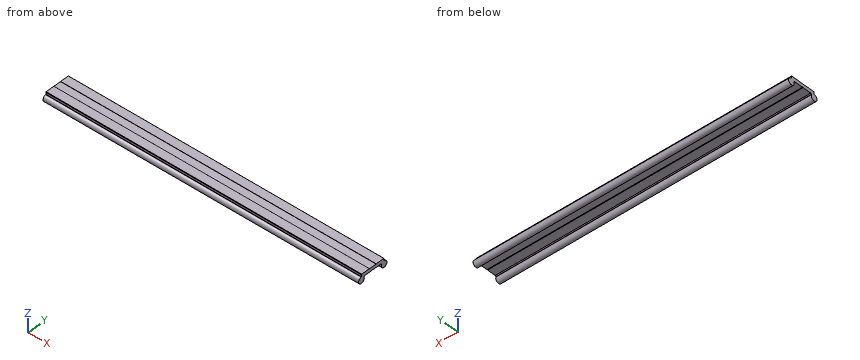
Autodesk Inventor part; units mm, degrees
ref_plane "YZ Plane" through (0, 0, 0) normal (1, 0, 0) x (0, 1, 0)
ref_plane "XZ Plane" through (0, 0, 0) normal (0, 1, 0) x (-1, 0, 0)
ref_plane "XY Plane" through (0, 0, 0) normal (0, 0, 1) x (1, 0, 0)
sketch "Szkic1" plane through (0, 0, 0) normal (1, 0, 0) x (0, 1, 0)
  line L0 (13.7, -0.2) -> (25.3, -0.2)
  line L1 (13.5, 0) -> (13.7, -0.2)
  line L2 (0, 0) -> (13.5, 0)
  line L3 (-0.5, -0.5) -> (0, 0)
  line L4 (-0.5, -3.7085) -> (-0.5, -0.5)
  arc A0 (-0.783, -4.008) -> (-0.5, -3.7085) centre (-0.8, -3.7085) ccw
  arc A1 (-0.783, -4.008) -> (3.9514, -6.7229) centre (-0.5, -9) ccw
  arc A2 (4.0685, -6.3265) -> (3.9514, -6.7229) centre (4.2185, -6.5863) ccw
  line L5 (5.5, -5.5) -> (4.0685, -6.3265)
  line L6 (19, -5.5) -> (5.5, -5.5)
  line L7 (19.5, -5.2113) -> (19, -5.5)
  line L8 (20, -5.5) -> (19.5, -5.2113)
  line L9 (33.5, -5.5) -> (20, -5.5)
  line L10 (34.9315, -6.3265) -> (33.5, -5.5)
  arc A3 (35.0486, -6.7229) -> (34.9315, -6.3265) centre (34.7815, -6.5863) ccw
  arc A4 (35.0486, -6.7229) -> (39.783, -4.008) centre (39.5, -9) ccw
  arc A5 (39.5, -3.7085) -> (39.783, -4.008) centre (39.8, -3.7085) ccw
  line L11 (39.5, -0.5) -> (39.5, -3.7085)
  line L12 (39, 0) -> (39.5, -0.5)
  line L13 (25.5, 0) -> (39, 0)
  line L14 (25.3, -0.2) -> (25.5, 0)
  point P0 (19.5, 0)
extrude "Wyciągnięcie proste1" add sketch "Szkic1" along normal blind 500
properties part number "WS_10_40_Z" material "Stal nierdzewna"
Source: CAD feature listing. Evaluate the final solid. Frame: model axes, mm. Round coordinates to 2 decimals unless told otherwise and drop trailing zeros. Order: outer loops, then holes, each group sorted by start corner. A loop starts at its lowest first (then second) coordinate and runs counter-clockwise, first axis right, second up. Notation, with made-up numbers: (-25, 82.5) -> (15, 82.5) arc R32 cw to (15, 113.5) -> close; hole circle Ø7 at (-0.75, 37.5). An arc over 180 degrees is marked (long way). One line per item, written item: value. Start each with the question number.
Q1. Section query B-B (x = 79.5). Return the cut outline in (y, z), plus the area to 3 significant figures.
Q2. Pin query (flat end, axial travel): pin 1 (3 mm diameter, centred on x = 380.5, y = 21.5, fed in from +Z); pin 2 (8 mm diameter, centred on x = 322.5, z = -2, fed in from +Y); pin 3 (1 mm diameter, centred on x = 194, z = -3, fed in from -Y). Return the tip coordinate at first contact, or that it passes through.
Q3. Section query A-A (z = -9). Return the cut outline in (x, y).
Q4. Material intervals for probe 1 along Y at (x, z) = (72.5, -8.25); probe 2 along Y at (x, z) = (186, -7.75); probe 3 along Z at (x, y) = (140, 16), sorted ascending.
Findings below:
1. outline: (-0.78, -4.01) arc R5 ccw (long way) to (3.95, -6.72) arc R0.3 cw to (4.07, -6.33) -> (5.5, -5.5) -> (19, -5.5) -> (19.5, -5.21) -> (20, -5.5) -> (33.5, -5.5) -> (34.93, -6.33) arc R0.3 cw to (35.05, -6.72) arc R5 ccw (long way) to (39.78, -4.01) arc R0.3 cw to (39.5, -3.71) -> (39.5, -0.5) -> (39, 0) -> (25.5, 0) -> (25.3, -0.2) -> (13.7, -0.2) -> (13.5, 0) -> (0, 0) -> (-0.5, -0.5) -> (-0.5, -3.71) arc R0.3 cw to start
1. area: 369 mm²
2. pin 1: z = -0.2
2. pin 2: y = 43.5
2. pin 3: y = -0.5
3. outline: (0, -5.5) -> (500, -5.5) -> (500, 4.5) -> (0, 4.5) -> close; (0, 34.5) -> (500, 34.5) -> (500, 44.5) -> (0, 44.5) -> close
4. probe 1: -5.44 to 4.44, 34.56 to 44.44
4. probe 2: -5.34 to 4.34, 34.66 to 44.34
4. probe 3: -5.5 to -0.2
